```python
from build123d import *

# Parameters (mm, degrees)
SKETCH1_R                = 16.5
BOSS_EXTRUDE1_DEPTH      = 130
BOSS_EXTRUDE2_DEPTH      = 5
BOSS_EXTRUDE2_DEPTH_BACK = 5
SKETCH3_R                = 6.5
CUT_EXTRUDE1_DEPTH       = 20


with BuildPart() as part:
    # Sketch1 → Boss-Extrude1 (new body)
    with BuildSketch(Plane.XY):
        Circle(SKETCH1_R)
    extrude(amount=BOSS_EXTRUDE1_DEPTH)

    # Sketch2 → Boss-Extrude2 (add, two sides: drawn at the far end of the back side and taken through both)
    with BuildSketch(Plane(origin=(0, 0, 0), x_dir=(1, 0, 0), z_dir=(0, 1, 0)).offset(-BOSS_EXTRUDE2_DEPTH_BACK)):
        Polygon((0, -98.214285714), (122.285351257, -185.560965183), (138.560020681, -162.77642799), (0, -63.804984646), align=None)
    extrude(amount=BOSS_EXTRUDE2_DEPTH + BOSS_EXTRUDE2_DEPTH_BACK)

    # Sketch3 → Cut-Extrude1 (cut)
    with BuildSketch(Plane(origin=(0, 5, 0), x_dir=(1, 0, 0), z_dir=(0, 1, 0))):
        with Locations(Location((117.40295043, -164.868885487, 0), (0, 0, 270))):
            Circle(SKETCH3_R)
    extrude(amount=-CUT_EXTRUDE1_DEPTH, mode=Mode.SUBTRACT)


solid = part.part
```
The model under review builds one solid part; all positions refer to its coordinate system, in mm. A direction names the side the tool comes from. Round coordinates to 2 decimals unless told otherwise and drop trailing zeros. Order: outer loops, then holes, each group sorted by start corner. A loop starts at its lowest first (then second) coordinate and runs counter-clockwise, first axis right, second up. Notation, with made-up numbers: (-21, 9.5) -> (-17, 9.5) arc R38 cw to (-17, 48.5) -> close; hole circle Ø7 at (2, 71.5). An arc over 180 degrees is marked (long way). One line per item, written item: value. Start each with the question number.
Q1. Machinability: for faces 4 (the face through (0, 0, 130)), 5 (the face through (72, 5, 134)), 6 (the face through (68.3, -0.1, 147)), which of the approach directions +Z, -Z, +X, -X, +Y, -Y give a long, thin tool a straight path to every point of the face, cutting with its end or side? Answer none if there is none.
Q2. Wall thickness on line 1 (Y direction, x = 131, z = 168); line 2 (Z direction, x = 2.5, y = -1.5); line 3 (X direction, y = 7, z = 43.5): over which ranges is each line inside the solid? List them lowest first.
Q3. Take a section at C-C (z = 167.5). Write out the cut boundary in (x, y).
Q4. Clearance check with flat-ended pins moving along their axes: pin 1 Ø2 at (y, z) = (-11, 48.5) entering from +X; pin 2 Ø5 at (y, z) = (11.5, 89) entering from -X; pin 3 Ø8 at (x, y) = (20.5, -8.5) entering from -Z. State where each tip first meets the part, or that it passes through.
Q5. Take a section at D-D (z = 25). Write out the cut boundary in (x, y), and give its area (3 significant figures).
Q6. Mouldability with a two-part tool opening along X and no side actions: class faces 1 (the face through (130.309, -0.07, 174.328)), 2 (the face through (72, -5, 134)), 3 (the face through (117.689, 0.07, 158.375)) as released by +X, released by -X, zero draft, split by the parting line, or undercut.
Q7. Take a section at A-A (x = 115). Write out the cut boundary in (y, z).
Q8. Take a section at B-B (y = 0). Write out the cut boundary in (x, z).
Reported:
1. face 4: +Z, -X, +Y, -Y
1. face 5: +Z, -Z, +X, +Y
1. face 6: +Z, +Y, -Y
2. line 1: y = -5 to 5
2. line 2: z = 0 to 130
2. line 3: x = -14.94 to 14.94
3. outline: (97, -5) -> (111.46, -5) -> (111.46, 5) -> (97, 5) -> close; (123.35, -5) -> (135.19, -5) -> (135.19, 5) -> (123.35, 5) -> close
4. pin 1: stops at x = 13.12
4. pin 2: stops at x = -13.83
4. pin 3: stops at z = 77.06
5. outline: circle Ø33 at (0, 0)
5. area: 855 mm2
6. face 1: released by +X
6. face 2: zero draft
6. face 3: undercut
7. outline: (-5, 145.95) -> (5, 145.95) -> (5, 158.83) -> (-5, 158.83) -> close; (-5, 170.91) -> (5, 170.91) -> (5, 180.36) -> (-5, 180.36) -> close
8. outline: (-16.5, 0) -> (16.5, 0) -> (16.5, 75.59) -> (138.56, 162.78) -> (122.29, 185.56) -> (16.5, 110) -> (16.5, 130) -> (-16.5, 130) -> close; hole circle Ø13 at (117.4, 164.87)
